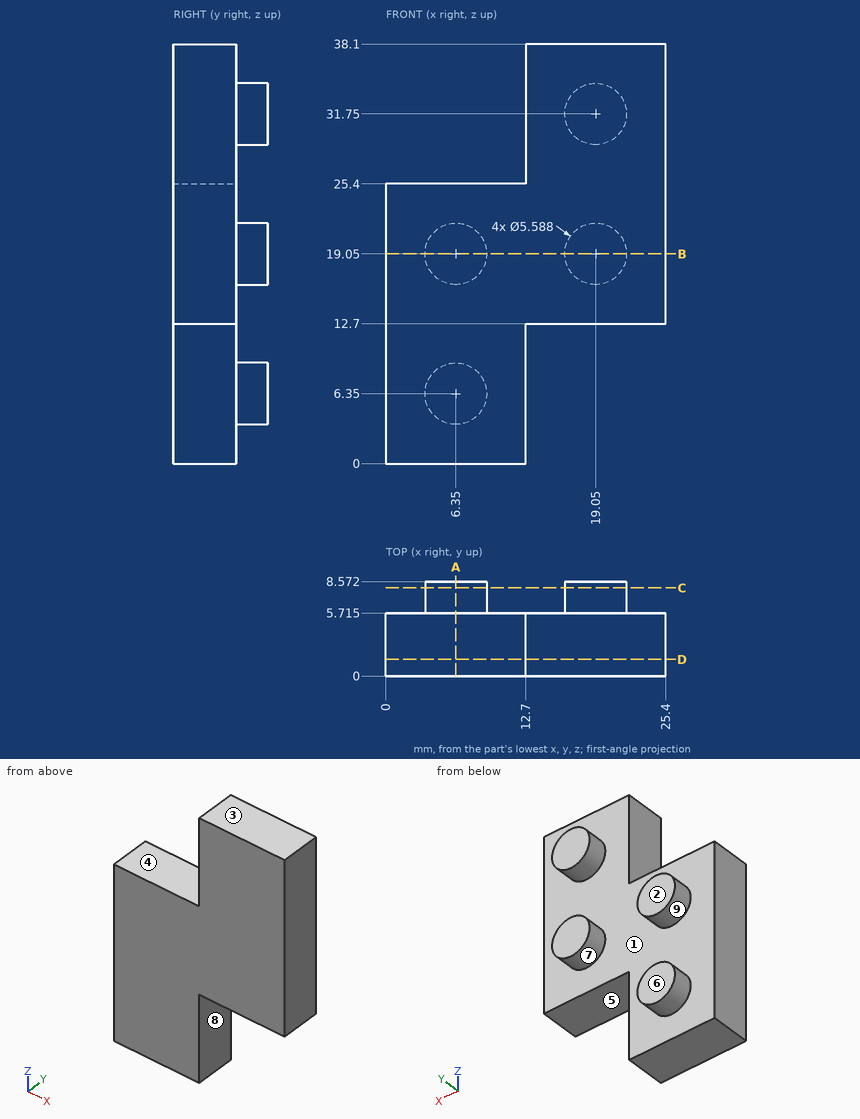
Study the drawing (mm; zero at the part's minimum x, y, z) and answer. A direction names the side the tool comes from. Give positions to 0.01 mm unless a question says otherwise; leave off trailing zeros. Loops run counter-clockwise (first coordinate to the right, second up) from the corner with the lowest first, then second, coordinate; pieces in that order, holes last. Notation, with made-up numbers: M 65,56.5 L 93,56.5 A19 ccw 93,89.5 Z; hole C 62.25,-12.75 d3. An arc over 180 degrees is marked long. One line per item, written item: value.
1. For the marked faces 1, 2, 3, 4 and 5, determine the directions among +Z, -Z, +X, -X, +Y, -Y from which every point of the face is accessible in a straight line to the end or side of a thin tool.
Found:
face 1: +Y
face 2: +Z, -Z, +X, -X, +Y
face 3: +Z, +X, -X, +Y, -Y
face 4: +Z, -X, +Y, -Y
face 5: -Z, +X, +Y, -Y
2. Find the intervals of material crossed by probe 1 along Y at (x, z) = (10, 24) (1 decimal); probe 2 along Z at (x, y) = (12.75, 1); probe 3 along Z at (x, y) = (11.75, 2), in increasing order.
Found:
probe 1: 0 to 5.7
probe 2: 12.7 to 38.1
probe 3: 0 to 25.4
3. Section B-B on z = 19.05 is taken. Determine the outline of the cut face in (x, y) (1 decimal).
Found:
outline: M 0,0 L 25.4,0 L 25.4,5.7 L 21.8,5.7 L 21.8,8.6 L 16.3,8.6 L 16.3,5.7 L 9.1,5.7 L 9.1,8.6 L 3.6,8.6 L 3.6,5.7 L 0,5.7 Z
4. Section C-C on y = 8 is taken. State how many separate pieces and enclosed holes the cut face has.
Found:
separate pieces: 4
enclosed holes: 0
5. For a pull along X with two mould halves and no side action, classify the marked faces 6, 7, 8 and 9 as pulls with the +X half, pulls with the -X half, needs draft (parallel to the pull), parting line crosses it, or undercut.
Found:
face 6: needs draft
face 7: undercut
face 8: pulls with the +X half
face 9: undercut
6. Section D-D on y = 1.5 is taken. Determine the outline of the cut face in (x, z).
Found:
outline: M 0,0 L 12.7,0 L 12.7,12.7 L 25.4,12.7 L 25.4,38.1 L 12.7,38.1 L 12.7,25.4 L 0,25.4 Z
7. Each of these flat-tipped pins is pushed along its axis until it touches: P1, Ø1.7, axis at y = 4, z = 8, coming from the +X side; P2, Ø4.5, axis at x = 17, y = 4, coming from the -Z side; P3, Ø4.5, axis at x = 9.5, y = 1.5, coming from the +Z side. Where does it stop, or does it pass through?
Found:
P1: x = 12.7
P2: z = 12.7
P3: z = 25.4
8. Section A-A on x = 6.35 is taken. Determine the outline of the cut face in (y, z) (1 decimal).
Found:
outline: M 0,0 L 5.7,0 L 5.7,3.6 L 8.6,3.6 L 8.6,9.1 L 5.7,9.1 L 5.7,16.3 L 8.6,16.3 L 8.6,21.8 L 5.7,21.8 L 5.7,25.4 L 0,25.4 Z
